Design review of the part built by this model. Coordinates are the model's own, in mm. Face numbers are marked on the shaded views. A direction names the side the tool comes from. Give positions to 0.01 mm unless a question says otherwise; leave off trailing zeros. Loops run counter-clockwise (first coordinate to the right, second up) from the corner with the lowest first, then second, coordinate; pieces in that order, holes last. Notation, with made-up numbers: (-2.5, -8.5) -> (37.5, -8.5) arc R27 ccw to (37.5, 11.5) -> close; hole circle Ø4 at (-7.75, 76.25). An arc over 180 degrees is marked (long way). Use a Markdown table: item, result. Add a question column.
1. Draft analysis for pull direction Z (two halves, no side actions). For the marked faces 1, 2, 3 and 4, state which applies: pulls with the +Z half, pulls with the -Z half, needs draft (parallel to the pull), parting line crosses it, or undercut.
2. To check wall thickness, follow line 1 (X direction, y = 1.45, z = 10); line 2 (X direction, y = 16.4, z = -18.75); line 3 (Z direction, x = 0, y = 2.6). State the ranges of each line that lie inside material, in increasing order.
3. For pin 1 Ø6 at (x, y) = (-18.5, 3) entering from +Z; pin 2 Ø10 at (x, z) = (-3, 22) entering from +Y; pin 3 Ø3.5 at (x, y) = (-7.5, 16) entering from -Z; pin 4 Ø1 at (y, z) = (6, -15.5) entering from +X, all flat-tipped, find the tip position at first contact; note any pin that passes through.
4. Add section D-D (x = -19). State the section outline as (y, z) points.
5. Add section C-C (y = 7). State the section outline as (x, z) points.
6. Add section B-B (x = -10.5). State the section outline as (y, z) points.
7. For the marked faces 5 and 6, list the 3-axis set-ups (+Z, -Z, +X, -X, +Y, -Y) from which the entire face can be reached by the end or side of a thin tool; tool diameter is ignored.
8. Add section A-A (z = 0). State the section outline as (x, y) points, and give its area (3 significant figures).
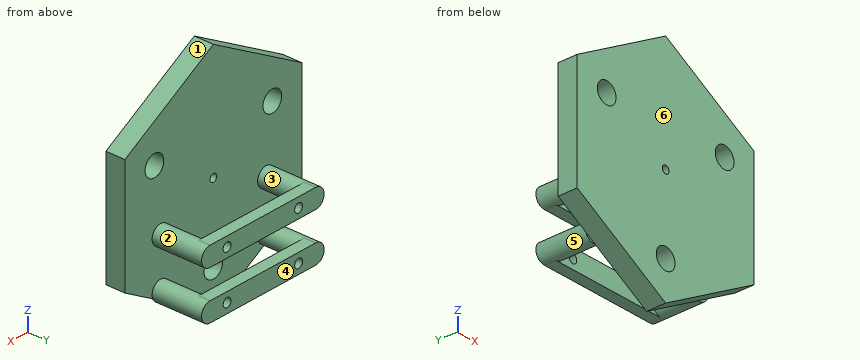
Autodesk Inventor part; units mm, degrees
ref_plane "YZ Plane" through (0, 0, 0) normal (1, 0, 0) x (0, 1, 0)
ref_plane "XZ Plane" through (0, 0, 0) normal (0, 1, 0) x (-1, 0, 0)
ref_plane "XY Plane" through (0, 0, 0) normal (0, 0, 1) x (1, 0, 0)
sketch "Sketch1" plane through (0, 0, 0) normal (0, 1, 0) x (-1, 0, 0)
  line L0 (0, 0) -> (0, -30)
  circle A0 centre (0, 0) radius 30
  line L1 (0, -30) -> (-25.9808, -15)
  line L2 (0, -30) -> (30, -30) construction
  line L3 (-25.9808, -15) -> (-25.9808, 15)
  line L4 (-25.9808, -15) -> (4.0192, -15) construction
  line L5 (-25.9808, 15) -> (0, 30)
  line L6 (0, 30) -> (25.9808, 15)
  line L7 (25.9808, 15) -> (25.9808, -15)
  line L8 (0, -30) -> (25.9808, -15)
  dimension "d0" = 30
  dimension "d1" = 150
  dimension "d3" = 30
  dimension "d4" = 90
  dimension "d5" = 30
  dimension "d6" = 120
  dimension "d7" = 25.9808
extrude "Extrusion1" add sketch "Sketch1" along normal blind 5 contours L7 L8 L1 L3 L5 L6
sketch "Sketch2" plane through (0, 5, 0) normal (0, 1, 0) x (1, 0, 0)
  line L0 (0, 0) -> (0, 20)
  circle A0 centre (0, 20) radius 2.75
  line L1 (0, 0) -> (17.3205, -10)
  line L2 (0, 0) -> (20, 0) construction
  line L3 (0, 0) -> (-17.3205, -10)
  line L4 (0, 0) -> (20, 0) construction
  circle A1 centre (-17.3205, -10) radius 2.75
  circle A2 centre (17.3205, -10) radius 2.75
  dimension "d10" = 20
  dimension "d11" = 5.5
  dimension "d12" = 20
  dimension "d13" = 30
  dimension "d14" = 20
  dimension "d15" = 150
  dimension "d16" = 5.5
  dimension "d17" = 5.5
extrude "Extrusion2" cut sketch "Sketch2" against normal blind 10
sketch "Sketch3" plane through (0, 5, 0) normal (0, 1, 0) x (1, 0, 0)
  line L0 (0, 0) -> (0, 12.5)
  line L1 (10.5, 6.25) -> (-10.5, 6.25)
  line L2 (-10.5, 6.25) -> (-10.5, 18.75)
  line L3 (-10.5, 18.75) -> (10.5, 18.75)
  line L4 (10.5, 18.75) -> (10.5, 6.25)
  line L5 (10.5, 6.25) -> (-10.5, 18.75) construction
  line L6 (-10.5, 6.25) -> (10.5, 18.75) construction
  line L7 (-10.5, 18.75) -> (-15.5, 18.75)
  line L8 (-10.5, 6.25) -> (-15.5, 6.25)
  line L9 (10.5, 18.75) -> (15.5, 18.75)
  line L10 (10.5, 18.75) -> (15.5, 18.75) construction
  line L11 (10.5, 6.25) -> (15.5, 6.25)
  circle A0 centre (-15.5, 18.75) radius 2.5
  circle A1 centre (-15.5, 6.25) radius 2.5
  circle A2 centre (15.5, 18.75) radius 2.5
  circle A3 centre (15.5, 6.25) radius 2.5
  dimension "d20" = 12.5
  dimension "d21" = 21
  dimension "d22" = 12.5
  dimension "d29" = 5
  dimension "d30" = 5
  dimension "d31" = 5
  dimension "d32" = 0
  dimension "d33" = 5
  dimension "d34" = 5
  dimension "d35" = 5
  dimension "d36" = 5
  dimension "d37" = 5
extrude "Extrusion4" add sketch "Sketch3" along normal blind 10 contours A1 | A0 | A2 | A3
sketch "Sketch4" plane through (-15.5, 15, -18.75) normal (0, 1, 0) x (1, 0, 0)
  circle A0 centre (0, 0) radius 2.5
  line L0 (0, 2.5) -> (31, 2.5)
  line L1 (31, 2.5) -> (31, -2.5)
  line L2 (31, -2.5) -> (0, -2.5)
  line L3 (0, -2.5) -> (0, 2.5)
  circle A1 centre (0, -12.5) radius 2.5
  line L4 (0, -10) -> (31, -10)
  line L5 (31, -10) -> (31, -15)
  line L6 (31, -15) -> (0, -15)
  line L7 (0, -15) -> (0, -10)
  circle A2 centre (31, -12.5) radius 2.5
  circle A3 centre (31, 0) radius 2.5
  point P0 (15.5, -18.75)
  dimension "d40" = 31
  dimension "d41" = 5
  dimension "d42" = 2.5
  dimension "d43" = 31
  dimension "d44" = 5
  dimension "d49" = 2.5
extrude "Extrusion5" add sketch "Sketch4" along normal blind 3
sketch "Sketch5" plane through (-15.5, 18, -18.75) normal (0, 1, 0) x (1, 0, 0)
  circle A0 centre (0, 0) radius 2.5
  line L0 (0, 0) -> (5, 0)
  arc A1 (31, -2.5) -> (31, 2.5) centre (31, 0) ccw
  line L1 (31, 0) -> (26, 0)
  circle A2 centre (0, -12.5) radius 2.5
  line L2 (0, -12.5) -> (5, -12.5)
  circle A3 centre (31, -12.5) radius 2.5
  line L3 (31, -12.5) -> (26, -12.5)
  circle A4 centre (5, 0) radius 1.15
  circle A5 centre (26, 0) radius 1.15
  circle A6 centre (5, -12.5) radius 1.15
  circle A7 centre (26, -12.5) radius 1.15
  point P0 (15.5, -18.75)
  dimension "d52" = 5
  dimension "d53" = 5
  dimension "d54" = 5
  dimension "d55" = 5
  dimension "d56" = 2.3
  dimension "d57" = 2.3
  dimension "d58" = 2.3
  dimension "d59" = 2.3
extrude "Extrusion6" cut sketch "Sketch5" against normal blind 3 contours A4 | A6 | A7 | A5
sketch "Sketch6" plane through (0, 5, 0) normal (0, 1, 0) x (1, 0, 0)
  circle A0 centre (0, 0) radius 1
  dimension "d62" = 2
extrude "Extrusion7" cut sketch "Sketch6" against normal blind 10
properties part number "80_20_Connector_Bot"
Taken from the geometry:
| question | item | result |
|---|---|---|
| 1 | face 1 | pulls with the +Z half |
| 1 | face 2 | undercut |
| 1 | face 3 | undercut |
| 1 | face 4 | needs draft |
| 2 | line 1 | x = -25.98 to -20.07, -14.57 to 14.57, 20.07 to 25.98 |
| 2 | line 2 | x = -18 to -11.65, -9.35 to 9.35, 11.65 to 18 |
| 2 | line 3 | z = -30 to -22.75, -17.25 to -1, 1 to 30 |
| 3 | pin 1 | stops at z = 21.05 |
| 3 | pin 2 | stops at y = 5 |
| 3 | pin 3 | stops at z = -21.25 |
| 3 | pin 4 | passes through |
| 4 | outline | (0, -19.03) -> (5, -19.03) -> (5, 7.82) -> (0, 7.82) -> close; (0, 12.18) -> (5, 12.18) -> (5, 19.03) -> (0, 19.03) -> close |
| 5 | outline | circle Ø5 at (-15.5, -18.75); circle Ø5 at (-15.5, -6.25); circle Ø5 at (15.5, -18.75); circle Ø5 at (15.5, -6.25) |
| 6 | outline | (0, -23.94) -> (5, -23.94) -> (5, 23.94) -> (0, 23.94) -> close; (15, -21.25) -> (18, -21.25) -> (18, -19.9) -> (15, -19.9) -> close; (15, -17.6) -> (18, -17.6) -> (18, -16.25) -> (15, -16.25) -> close; (15, -8.75) -> (18, -8.75) -> (18, -7.4) -> (15, -7.4) -> close; (15, -5.1) -> (18, -5.1) -> (18, -3.75) -> (15, -3.75) -> close |
| 7 | face 5 | none |
| 7 | face 6 | +Z, -Z, +X, -X, -Y |
| 8 | outline | (-25.98, 0) -> (-1, 0) -> (-1, 5) -> (-25.98, 5) -> close; (1, 0) -> (25.98, 0) -> (25.98, 5) -> (1, 5) -> close |
| 8 | area | 250 mm^2 |
